Print and shaded views of the part. All mm, measured from the part's lowest x, y and z. Give positions to 0.01 mm unless a question says otherwise; leave off trailing zeros. Loops run counter-clockwise (first coordinate to the right, second up) from the corner with the lowest first, then second, coordinate; pieces in that order, holes last.
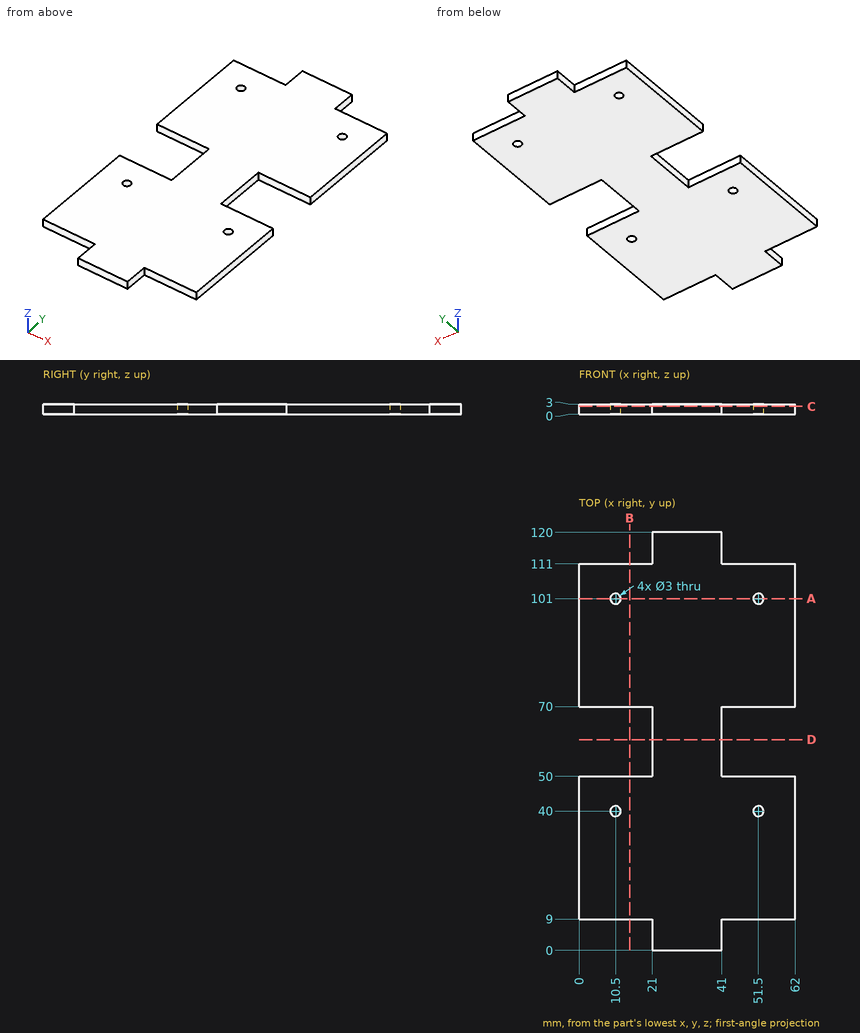
1. Saw through at B-B, the plane x = 14.5. List the corners of the cut face in (y, z), and give its area (3 significant figures).
Responses:
outline: (9, 0) - (50, 0) - (50, 3) - (9, 3) - close; (70, 0) - (111, 0) - (111, 3) - (70, 3) - close
area: 246 mm2
2. Saw through at A-A, the plane y = 101. List the corners of the cut face in (x, z).
Responses:
outline: (0, 0) - (9, 0) - (9, 3) - (0, 3) - close; (12, 0) - (50, 0) - (50, 3) - (12, 3) - close; (53, 0) - (62, 0) - (62, 3) - (53, 3) - close
3. Saw through at D-D, the plane y = 60.5. List the corners of the cut face in (x, z), and give its area (3 significant figures).
Responses:
outline: (21, 0) - (41, 0) - (41, 3) - (21, 3) - close
area: 60.0 mm2
4. Saw through at C-C, the plane z = 2.3. List the corners of the cut face in (x, y).
Responses:
outline: (0, 9) - (21, 9) - (21, 0) - (41, 0) - (41, 9) - (62, 9) - (62, 50) - (41, 50) - (41, 70) - (62, 70) - (62, 111) - (41, 111) - (41, 120) - (21, 120) - (21, 111) - (0, 111) - (0, 70) - (21, 70) - (21, 50) - (0, 50) - close; hole circle Ø3 at (10.5, 40); hole circle Ø3 at (10.5, 101); hole circle Ø3 at (51.5, 40); hole circle Ø3 at (51.5, 101)
5. Drop flat-ended pins along their axis: pin 1 (0.9 mm diameter, centred on x = 49.5, z = 2, fed in from +Y); pin 2 (0.9 mm diameter, centred on y = 55.5, z = 1, fed in from -X); pin 3 (0.9 mm diameter, centred on x = 9, z = 1.5, fed in from -Y). Give the stop position or say it passes through.
Responses:
pin 1: stops at y = 111
pin 2: stops at x = 21
pin 3: stops at y = 9
6. Probe line 1 along Y through (x, z) = (51.5, 0.75); line 2 along X through (y, z) = (101, 1.35); line 3 along Y through (x, z) = (59, 1.45). List the from-to ranges inside material, lowest first.
Responses:
line 1: y = 9 to 38.5, 41.5 to 50, 70 to 99.5, 102.5 to 111
line 2: x = 0 to 9, 12 to 50, 53 to 62
line 3: y = 9 to 50, 70 to 111
